For this review, use the dimensioned drawing (mm, ordinates from the lowest corner) and the shaded views. Round coordinates to 2 decimals unless told otherwise and drop trailing zeros. Order: outer loops, then holes, each group sorted by start corner. A loop starts at its lowest first (then second) coordinate and runs counter-clockwise, first axis right, second up. Notation, with made-up numbers: (63.5, -20) -> (81.5, -20) arc R25 cw to (81.5, -7) -> close; hole circle Ø6 at (74, -2.75). An arc over 180 degrees is marked (long way). Answer in a Markdown table with one row per item.
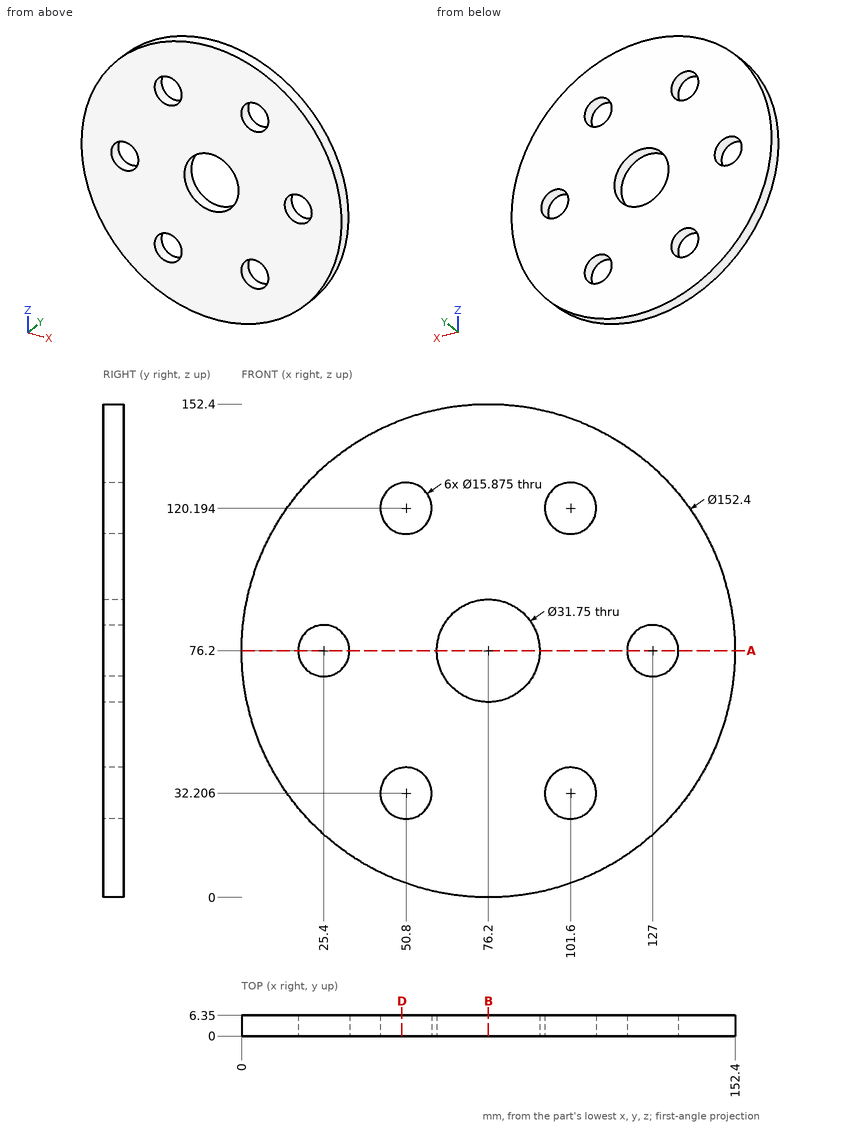
Q1. Clearance check with flat-ended pins moving along their axes: pin 1 Ø3 at (y, z) = (5.5, 85.5) entering from +X; pin 2 Ø1.5 at (x, y) = (39, 1.5) entering from +Z; pin 3 Ø9.5 at (x, z) = (101.6, 120.19) entering from -Y; pin 4 Ø1.5 at (y, z) = (1.5, 121) entering from -X. State where each tip first meets the part, or that it passes through.
Answer key:
| item | result |
|---|---|
| pin 1 | stops at x = 152 |
| pin 2 | stops at z = 143.12 |
| pin 3 | passes through |
| pin 4 | stops at x = 14.02 |
Q2. Take a section at A-A, the plane z = 76.2. Give the number of separate pieces and of enclosed holes in the cut face.
Answer key:
| item | result |
|---|---|
| separate pieces | 4 |
| enclosed holes | 0 |
Q3. To check wall thickness, follow probe 1 along X at (y, z) = (6, 113) (1 decimal); probe 2 along Z at (x, y) = (101.6, 4.5); probe 3 along X at (y, z) = (5, 79). State the ranges of each line that lie inside material, in increasing order.
Answer key:
| item | result |
|---|---|
| probe 1 | x = 9.5 to 47.4, 54.2 to 98.2, 105 to 142.9 |
| probe 2 | z = 4.36 to 24.27, 40.14 to 112.26, 128.13 to 148.04 |
| probe 3 | x = 0.05 to 17.97, 32.83 to 60.57, 91.83 to 119.57, 134.43 to 152.35 |
Q4. Take a section at D-D, the plane x = 49.5. Write out the cut boundary in (y, z).
Answer key:
| item | result |
|---|---|
| outline | (0, 4.83) -> (6.35, 4.83) -> (6.35, 24.38) -> (0, 24.38) -> close; (0, 40.04) -> (6.35, 40.04) -> (6.35, 112.36) -> (0, 112.36) -> close; (0, 128.02) -> (6.35, 128.02) -> (6.35, 147.57) -> (0, 147.57) -> close |
Q5. Take a section at B-B, the plane x = 76.2. Write out the cut boundary in (y, z) (3 decimals), then the cut area to 3 significant figures.
Answer key:
| item | result |
|---|---|
| outline | (0, 0) -> (6.35, 0) -> (6.35, 60.325) -> (0, 60.325) -> close; (0, 92.075) -> (6.35, 92.075) -> (6.35, 152.4) -> (0, 152.4) -> close |
| area | 766 mm^2 |
